The model under review builds one solid part; all positions refer to its coordinate system, in mm. Round coordinates to 2 decimals unless told otherwise and drop trailing zeros. Loops run counter-clockwise (first coordinate to the right, second up) from the corner with the lowest first, then second, coordinate; pieces in that order, holes last. Notation, with made-up numbers: M 40.25,-21.5 L 67.25,-21.5 A15 cw 67.25,-17.5 Z; hole C 13.5,-27.5 d4. An arc over 180 degrees is marked long. One line per question, with ' | ' between items.
from build123d import *

# Parameters (mm, degrees)
SKETCH1_R                       = 7.62
BOSS_EXTRUDE1_DEPTH             = 6.35
F_5_0MM_DOWEL_HOLE1_D           = 5
F_5_0MM_DOWEL_HOLE1_CSINK_D     = 5.05
F_5_0MM_DOWEL_HOLE1_CSINK_ANGLE = 90
BOSS_EXTRUDE3_DEPTH             = 6.35
FILLET2_DEPTH                   = 6.35
F_5_0MM_DOWEL_HOLE3_D           = 5


with BuildPart() as part:
    # Sketch1 → Boss-Extrude1 (new body)
    with BuildSketch(Plane.XY):
        with BuildLine():
            ThreePointArc((-50.301924176, 44.54348243), (-52.533770503, 39.155328757), (-57.921924176, 36.92348243))
            Line((-57.921924176, 36.92348243), (43.628363104, 36.92348243))
            Line((43.628363104, 36.92348243), (82.81675676, -2.264911225))
            Line((82.81675676, -2.264911225), (145.132424058, -2.264911225))
            Line((145.132424058, -2.264911225), (102.962916525, 20.595088775))
            Line((102.962916525, 20.595088775), (102.962916525, 12.975088775))
            Line((102.962916525, 12.975088775), (89.12937145, 12.975088775))
            Line((89.12937145, 12.975088775), (49.940977795, 52.16348243))
            Line((49.940977795, 52.16348243), (-57.921924176, 52.16348243))
            ThreePointArc((-57.921924176, 52.16348243), (-52.533770503, 49.931636103), (-50.301924176, 44.54348243))
        make_face()
        with Locations((-57.921924176, 44.54348243)):
            Circle(SKETCH1_R)
    extrude(amount=BOSS_EXTRUDE1_DEPTH)

    # Ø5.0mm Dowel Hole1 (through all)
    with Locations(Plane.XY.offset(6.35)):
        with Locations((-57.921924176, 44.54348243)):
            CounterSinkHole(F_5_0MM_DOWEL_HOLE1_D / 2, F_5_0MM_DOWEL_HOLE1_CSINK_D / 2, counter_sink_angle=F_5_0MM_DOWEL_HOLE1_CSINK_ANGLE)

    # Sketch4 → Boss-Extrude3 (add)
    with BuildSketch(Plane.XY):
        with BuildLine():
            Line((-45.049324905, 52.16348243), (-35.049324905, 52.16348243))
            Line((-35.049324905, 52.16348243), (-35.049324905, 54.86223243))
            ThreePointArc((-35.049324905, 54.86223243), (-40.049324905, 59.86223243), (-45.049324905, 54.86223243))
            Line((-45.049324905, 54.86223243), (-45.049324905, 52.16348243))
        make_face()
    extrude(amount=BOSS_EXTRUDE3_DEPTH)

    # Fillet2: read off the stored shape, not the designer's step
    # Fillet2 outline → Fillet2 (add)
    with BuildSketch(Plane.XY):
        with BuildLine():
            Line((-35.049324905, 52.16348243), (-30.317714122, 52.16348243))
            add(Edge.make_bspline(
                [(-30.317714122, 52.16348243), (-31.005571174, 52.16348243), (-31.693428226, 52.16348243), (-33.124030191, 52.387599223), (-34.337985858, 53.16866407), (-34.986310807, 54.947810993), (-35.077384253, 55.56402873), (-35.183519514, 56.01285743)],
                knots=[0, 0, 0, 0, 0, 0, 0.5, 0.5, 1, 1, 1, 1, 1, 1], degree=5))
            ThreePointArc((-35.183519514, 56.01285743), (-35.08298687, 55.441444413), (-35.049324905, 54.86223243))
            Line((-35.049324905, 54.86223243), (-35.049324905, 52.16348243))
        make_face()
        with BuildLine():
            ThreePointArc((-45.049324905, 54.86223243), (-45.01566294, 55.441444413), (-44.915130297, 56.01285743))
            add(Edge.make_bspline(
                [(-44.915130297, 56.01285743), (-45.021265558, 55.56402873), (-45.112339003, 54.947810993), (-45.760663953, 53.16866407), (-46.97461962, 52.387599223), (-48.405221585, 52.16348243), (-49.093078637, 52.16348243), (-49.780935689, 52.16348243)],
                knots=[0, 0, 0, 0, 0, 0, 0.5, 0.5, 1, 1, 1, 1, 1, 1], degree=5))
            Line((-49.780935689, 52.16348243), (-45.049324905, 52.16348243))
            Line((-45.049324905, 52.16348243), (-45.049324905, 54.86223243))
        make_face()
    extrude(amount=FILLET2_DEPTH)

    # Ø5.0mm Dowel Hole3 (through all)
    with Locations(Plane.XY.offset(6.35)):
        with Locations((-40.049324905, 54.86223243)):
            Hole(F_5_0MM_DOWEL_HOLE3_D / 2)


solid = part.part
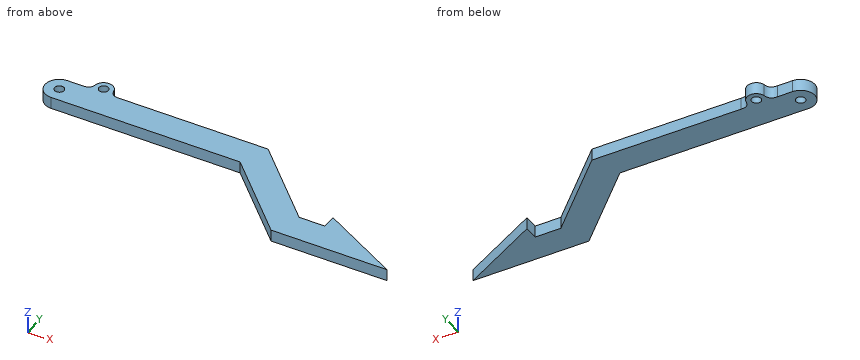
1) Add section C-C on y = 27.5. State the section outline as (x, z) points, then the cut area to 3 significant figures.
Output values:
outline: M 53.05,0 L 74.6,0 L 74.6,6.35 L 53.05,6.35 Z | area: 137 mm²
2) Add section B-B on z = 1.75. State how many separate pieces and enclosed holes the cut face has, then the cut area to 3 significant figures.
Output values:
separate pieces: 1 | enclosed holes: 2 | area: 3,310 mm²
3) Insertion check: P1, Ø3, axis at x = -19, z = 2.5, coming from the -Y side; P2, Ø1.9, axis at x = -52, z = 4, coming from the +Y side; P3, Ø1.5, axis at y = 41, z = 2, coming from the -X side. Each pin has a flat end and moves straight along its axis. Give the tip position at first contact, or say it passes through.
Output values:
P1: stops at y = 36.92 | P2: stops at y = 52.16 | P3: stops at x = -65.01
4) Add section A-A on x = 22. State the section outline as (y, z) points.
Output values:
outline: M 36.92,0 L 52.16,0 L 52.16,6.35 L 36.92,6.35 Z
5) For line 1 (Y direction, x = 15, z = 4); line 2 (X direction, y = 56, z = 2); line 3 (Y direction, x = 97.5, z = 0.5), list the stretches that pass through material, from the lowest coordinate up.
Output values:
line 1: y = 36.92 to 52.16 | line 2: x = -44.92 to -42.28, -37.82 to -35.18 | line 3: y = -2.26 to 12.98
